For this review, use the dimensioned drawing (mm, ordinates from the lowest corner) and the shaded views. Coordinates: 2 decimals unless noted, no trailing zeros. Write each loop counter-clockwise with the first axis right and the second up, starting at its lowest first coordinate (ties: lowest second). Pieces come first, ordered by that corner, then holes. Notation, with made-up numbers: (-23, 87.5) - (24, 87.5) arc R13 cw to (24, 104.5) - close; hole circle Ø2 at (43, 0.5). An arc over 180 degrees is marked (long way). One line per item, written item: value.
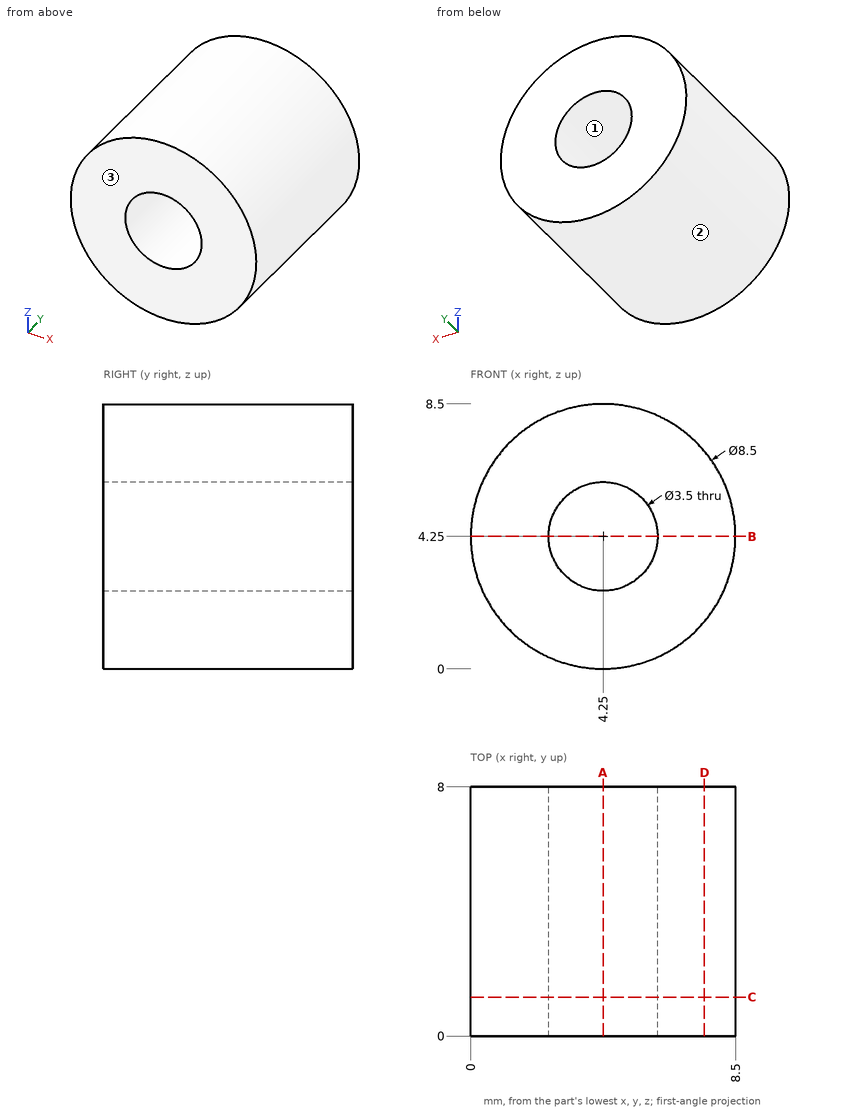
1. Insertion check: pin 1 Ø3 at (x, y) = (2.5, 1) entering from +Z; pin 2 Ø3 at (y, z) = (3, 7.5) entering from +X. Each pin has a flat end and moves straight along its axis. Give the tip position at first contact, or say it passes through.
Answer block:
pin 1: stops at z = 8.49
pin 2: stops at x = 8.12
2. Mouldability with a two-part tool opening along Z and no side actions: class the marked faces 1, 2 and 3 as released by +Z, released by -Z, zero draft, split by the parting line, or undercut.
Answer block:
face 1: undercut
face 2: split by the parting line
face 3: zero draft
3. Wall thickness on line 1 along X through (y, z) = (6.25, 4.25); line 2 along X through (y, z) = (0.5, 5.25): over which ranges is each line inside the solid? List them lowest first.
Answer block:
line 1: x = 0 to 2.5, 6 to 8.5
line 2: x = 0.12 to 2.81, 5.69 to 8.38
4. Consider section D-D, the plane x = 7.5. Write out the cut boundary in (y, z).
Answer block:
outline: (0, 1.51) - (8, 1.51) - (8, 6.99) - (0, 6.99) - close
5. Consider section C-C, the plane y = 1.25. Write out the cut boundary in (x, z).
Answer block:
outline: circle Ø8.5 at (4.25, 4.25); hole circle Ø3.5 at (4.25, 4.25)
6. Consider section A-A, the plane x = 4.25. Write out the cut boundary in (y, z).
Answer block:
outline: (0, 0) - (8, 0) - (8, 2.5) - (0, 2.5) - close; (0, 6) - (8, 6) - (8, 8.5) - (0, 8.5) - close
7. Consider section B-B, the plane z = 4.25. Write out the cut boundary in (x, y), then the cut area to 3 significant figures.
Answer block:
outline: (0, 0) - (2.5, 0) - (2.5, 8) - (0, 8) - close; (6, 0) - (8.5, 0) - (8.5, 8) - (6, 8) - close
area: 40.0 mm^2
